Can you work these out from the drawing? Everything is in mm from the part's minimum corner. A direction names the side the tool comes from. Round coordinates to 2 decimals unless told otherwise and drop trailing zeros. Order: outer loops, then holes, each group sorted by start corner. A loop starts at its lowest first (then second) coordinate and runs counter-clockwise, first axis right, second up. Notation, with made-up numbers: (69.5, 72) - (115.5, 72) arc R8 ccw to (115.5, 76) - close; hole circle Ø5 at (16.5, 65.5). An arc over 180 degrees is marked (long way). Write item = value, one per line.
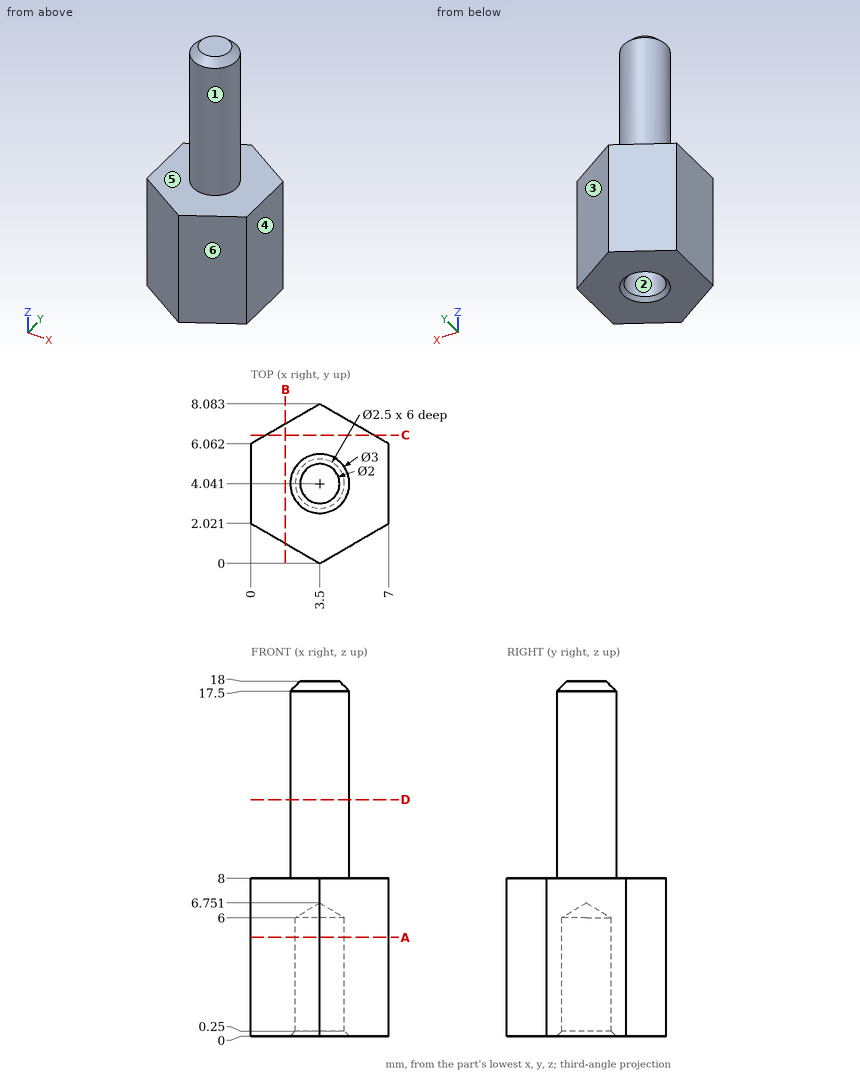
(1) If we section it at D-D (z = 12): Write out the boundary of the cut face in (x, y).
Computed:
outline = circle Ø3 at (3.5, 4.04)
(2) Thinking about a two-plate mould opening in Y: for the marked faces 1, 2, 3 and 4, which applies, +Y half, -Y half, draft (parallel to the pull), parting line (faces both ways), or undercut?
Computed:
face_1 = parting line
face_2 = undercut
face_3 = +Y half
face_4 = draft
(3) If we section it at C-C (y = 6.5): Write out the boundary of the cut face in (x, z).
Computed:
outline = (0.76, 0) - (6.24, 0) - (6.24, 8) - (0.76, 8) - close
(4) Will these pins go through, and if not, where does the flat tip stop? P1, Ø1.5, axis at y = 3.5, z = 16, coming from the -X side; P2, Ø4, axis at x = 3, z = 4.5, coming from the -Y side.
Computed:
P1 = 2
P2 = 0
(5) If we section it at B-B (x = 1.75): Write out the boundary of the cut face in (y, z).
Computed:
outline = (1.01, 0) - (7.07, 0) - (7.07, 8) - (1.01, 8) - close
(6) On a 3-axis mill with a long thin cutter (end or side, diameter ignored), from which of +Z, -Z, +X, -X, +Y, -Y can I reach the whole of each face in a straight line? I mean the marked faces 5 and 6. Say none if no direction works.
Computed:
face_5 = +Z
face_6 = +Z, -Z, +X, -Y
(7) If I drill on line 1 (Z direction, x = 5, y = 5); line 2 (X direction, y = 5, z = 3) (1 decimal); line 3 (X direction, y = 1.5, z = 5) (1 decimal), over which ranges is the centre line in solid material (lowest first)? Write a range as from..to.
Computed:
line_1 = 0..8
line_2 = 0..2.7, 4.3..7
line_3 = 0.9..6.1
(8) If we section it at A-A (z = 5): Write out the boundary of the cut face in (x, y).
Computed:
outline = (0, 2.02) - (3.5, 0) - (7, 2.02) - (7, 6.06) - (3.5, 8.08) - (0, 6.06) - close; hole circle Ø2.5 at (3.5, 4.04)
